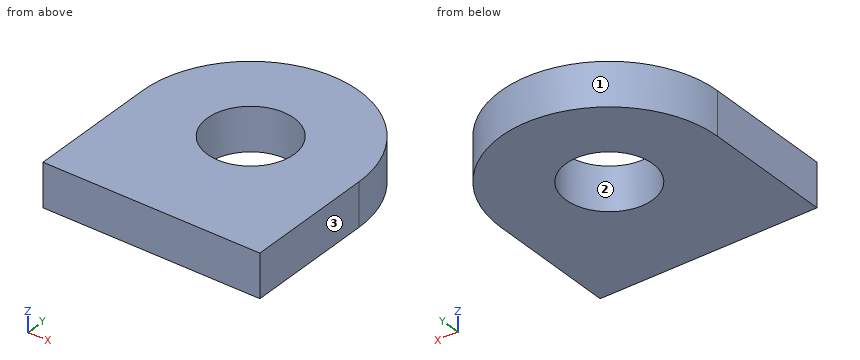
```python
from build123d import *

# Parameters (mm, degrees)
BOSS_EXTRUDE1_DEPTH = 10
SKETCH2_R           = 10
CUT_EXTRUDE1_DEPTH  = 10


with BuildPart() as part:
    # Sketch1 → Boss-Extrude1 (new body)
    with BuildSketch(Plane.XY):
        with BuildLine():
            Line((-25, 0), (-25, -30))
            Line((-25, -30), (25, -30))
            Line((25, -30), (25, 0))
            ThreePointArc((25, 0), (0, 25), (-25, 0))
        make_face()
    extrude(amount=BOSS_EXTRUDE1_DEPTH)

    # Sketch2 → Cut-Extrude1 (cut)
    with BuildSketch(Plane.XY.offset(10)):
        Circle(SKETCH2_R)
    extrude(amount=-CUT_EXTRUDE1_DEPTH, mode=Mode.SUBTRACT)


solid = part.part
```
Input: part model. Units: mm. Frame: model coordinates. Face numbers are marked on the shaded views. Round coordinates to 2 decimals unless told otherwise and drop trailing zeros. Loops run counter-clockwise (first coordinate to the right, second up) from the corner with the lowest first, then second, coordinate; pieces in that order, holes last. Notation, with made-up numbers: (74, -1.5) -> (127, -1.5) arc R32 cw to (127, 26.5) -> close; hole circle Ø7 at (-31, -24.5). An arc over 180 degrees is marked (long way). Use one line per item in the form item = value. Start each with the question number.
Item 1: Section query A-A on x = 0. Return the cut outline in (y, z).
Item 2: Section query D-D on y = 20.5. Return the cut outline in (x, z).
Item 3: Material intervals for L1, parallel to Y at x = 0, z = 6.5; L2, parallel to Y at x = -7.5, z = 1.25; L3, parallel to Y at x = 20, z = 6.75, sorted ascending. Write a range as from..to.
Item 4: Section query C-C on x = -5.5. Return the cut outline in (y, z).
Item 5: Contact query for flat-ended pins moving along their axis: pin 1 Ø5 at (y, z) = (3, 2) entering from -X (3 decimals); pin 2 Ø1 at (y, z) = (17.5, 3.5) entering from +X; pin 3 Ø16 at (x, y) = (0, 0) entering from -Z. Output: stop coordinate, or through.
Item 6: Section query B-B on z = 4. Return the cut outline in (x, y).
Item 7: Mould query, pull axis Y, two halves, no side actions, for the marked faces 1, 2 and 3. Classes: pulls with the +Y half, pulls with the -Y half, needs draft (parallel to the pull), parting line crosses it, or undercut.
Ans:
q1.outline = (-30, 0) -> (-10, 0) -> (-10, 10) -> (-30, 10) -> close; (10, 0) -> (25, 0) -> (25, 10) -> (10, 10) -> close
q2.outline = (-14.31, 0) -> (14.31, 0) -> (14.31, 10) -> (-14.31, 10) -> close
q3.L1 = -30..-10, 10..25
q3.L2 = -30..-6.61, 6.61..23.85
q3.L3 = -30..15
q4.outline = (-30, 0) -> (-8.35, 0) -> (-8.35, 10) -> (-30, 10) -> close; (8.35, 0) -> (24.39, 0) -> (24.39, 10) -> (8.35, 10) -> close
q5.pin_1 = -24.995
q5.pin_2 = 18.33
q5.pin_3 = through
q6.outline = (-25, -30) -> (25, -30) -> (25, 0) arc R25 ccw to (-25, 0) -> close; hole circle Ø20 at (0, 0)
q7.face_1 = pulls with the +Y half
q7.face_2 = undercut
q7.face_3 = needs draft
